Autodesk Inventor part; units mm, degrees
ref_plane "YZ Plane" through (0, 0, 0) normal (1, 0, 0) x (0, 1, 0)
ref_plane "XZ Plane" through (0, 0, 0) normal (0, 1, 0) x (-1, 0, 0)
ref_plane "XY Plane" through (0, 0, 0) normal (0, 0, 1) x (1, 0, 0)
sketch "Sketch1" plane through (0, 0, 0) normal (0, 1, 0) x (-1, 0, 0)
  line L0 (-125, 125) -> (125, 125)
  line L1 (125, 125) -> (125, -125)
  line L2 (125, -125) -> (-125, -125)
  line L3 (-125, -125) -> (-125, 125)
  line L4 (175, 0) -> (-175, 0) construction
  line L5 (0, -175) -> (0, 175) construction
  point P0 (0, 0)
  dimension "d0" = 250
  dimension "d1" = 250
extrude "Extrusion1" add sketch "Sketch1" along normal blind 3.175
sketch "Sketch2" plane through (0, 3.175, 0) normal (0, 1, 0) x (1, 0, 0)
  line L0 (0, 175) -> (0, -175) construction
  line L1 (175, 0) -> (-175, 0) construction
  line L2 (125, 125) -> (-125, 125)
  line L3 (60, -42.2089) -> (-60, -42.2089) construction
  line L4 (60, 45.5919) -> (-60, 45.5919) construction
  point P0 (0, 0)
  dimension "d4" = 79.4081
  dimension "d5" = 87.8008
  dimension "d6" = 120
hole "Hole1" at (60, 3.175, -45.5919) at (-60, 3.175, -45.5919) at (60, 3.175, 42.2089) at (-60, 3.175, 42.2089) direction (0, -1, 0) diameter 6 end through all
properties part number "Pedalbox_V2_Floor"
Geometry: final body of the model. Coordinates: model frame, mm. Give positions to 0.01 mm unless a question says otherwise; leave off trailing zeros. Order: outer loops, then holes, each group sorted by start corner. A loop starts at its lowest first (then second) coordinate and runs counter-clockwise, first axis right, second up. Notation, with made-up numbers: M 86.5,3 L 116.5,3 A5 cw 116.5,7 Z; hole C 83,23 d7. An arc over 180 degrees is marked long. Answer as CSV lines item,"result". Start each with the question number.
1) Mould query, pull axis X, two halves, no side actions, for faces 1 (the flat face through (2, 0, 2)), 2 (the cylindrical face through (-62.03, 1.57, -47.8)). Classes: +X half, -X half, draft (parallel to the pull), parting line (faces both ways), or undercut.
2) First-contact query: P1, Ø5.5, axis at x = 60, z = -45.59, coming from the +Y side; P2, Ø7, axis at x = -60, z = -45.59, coming from the -Y side. Flat tips, straight axial feed; report the tip coordinate or a pass-through.
3) Cut plane A-A (x = -60). Output: boundary loops of the cut face in (y, z) (3 decimals), then the cut area to 3 significant figures.
4) Line query: line 1 (Z direction, x = 60, y = 1.25); line 2 (X direction, y = 2.75, z = -43); line 3 (X direction, y = 0.65, z = -47). Output: solid intervals per line, ascending. Write a range as from..to.
Findings below:
1,face 1,"draft"
1,face 2,"undercut"
2,P1,"passes through"
2,P2,"stops at y = 0"
3,outline,"M 0,-125 L 3.175,-125 L 3.175,-48.592 L 0,-48.592 Z; M 0,-42.592 L 3.175,-42.592 L 3.175,39.209 L 0,39.209 Z; M 0,45.209 L 3.175,45.209 L 3.175,125 L 0,125 Z"
3,area,"756 mm²"
4,line 1,"z = -125..-48.59, -42.59..39.21, 45.21..125"
4,line 2,"x = -125..-61.51, -58.49..58.49, 61.51..125"
4,line 3,"x = -125..-62.65, -57.35..57.35, 62.65..125"
